Part print with two shaded views. Sizes in mm from the minimum x, y, z corner. A direction names the side the tool comes from. Give positions to 0.01 mm unless a question says otherwise; leave off trailing zeros. Order: outer loops, then holes, each group sorted by start corner. A loop starts at its lowest first (then second) coordinate and runs counter-clockwise, first axis right, second up. Notation, with made-up numbers: (-28.5, 16.25) -> (4.5, 16.25) arc R15 ccw to (4.5, 42.25) -> close; hole circle Ø10 at (85.25, -30.5). An arc over 180 degrees is marked (long way). Write item = value, one per line. Start each with the question number.
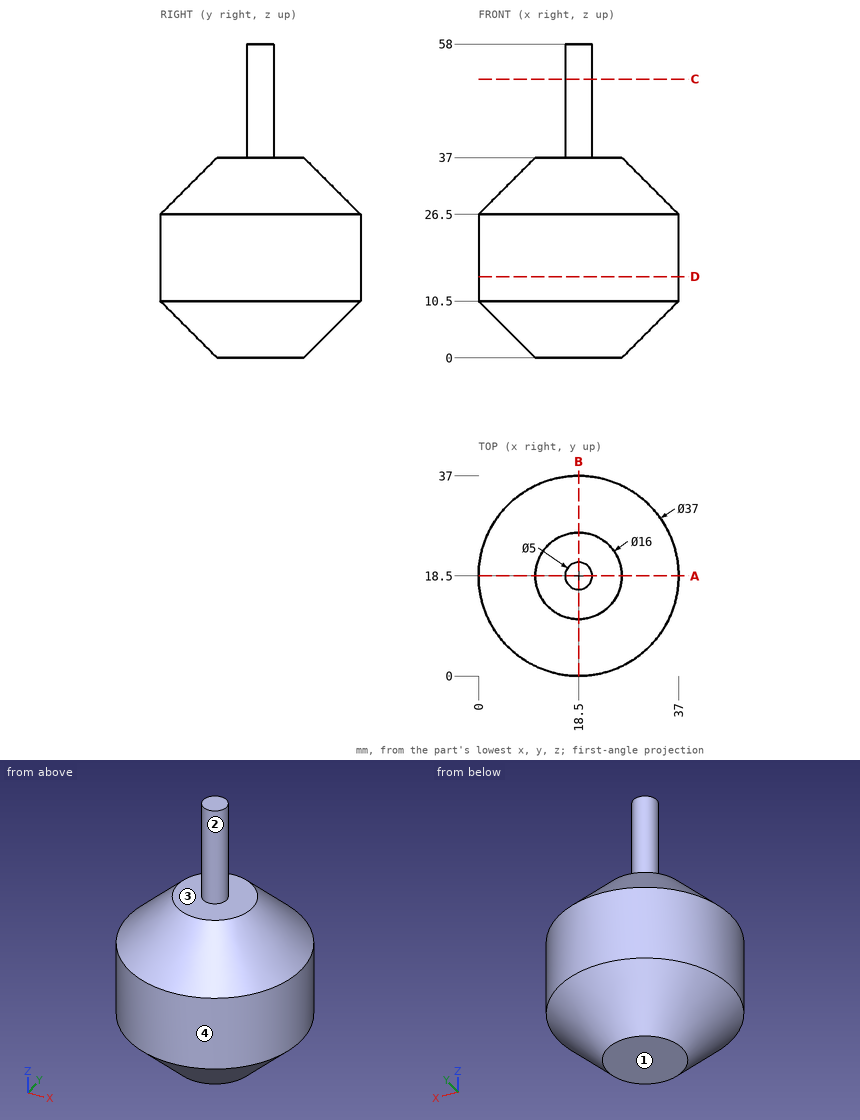
(1) Cut at C-C, the plane z = 51.5. Give the cut face in (x, y).
(2) Cut at A-A, the plane y = 18.5. Give the cut face in (x, z), plus the area to 3 significant figures.
(3) 3-axis set-ups, long thin cutter, end or side, ignore diameter. For the marked faces 1 and 2: which of +Z, -Z, +X, -X, +Y, -Y reach the whole face in a straight line?
(4) Wall check: line 1 (Y direction, x = 18, z = 11); line 2 (Z direction, x = 16.5, y = 23.5); line 3 (Z direction, x = 33, y = 27.5). Give the ranges that are in metal, low to high. Write a range as [from, to].
(5) Flat gauge pins, fed straight in: P1, Ø6, axis at x = 25, y = 31.5, coming from the +Z side; P2, Ø8, axis at x = 6, y = 4, coming from the -Z side; P3, Ø1.5, axis at x = 11, y = 20.5, coming from the +Z side. Where does each tip first touch, or does it go through?
(6) Cut at D-D, the plane z = 15. Give the cut face in (x, y).
(7) Mould opens along X. For the marked faces 3 and 4 say: released by +X, released by -X, zero draft, split by the parting line, or undercut.
Results:
q1.outline = circle Ø5 at (18.5, 18.5)
q2.outline = (0, 10.5) -> (10.5, 0) -> (26.5, 0) -> (37, 10.5) -> (37, 26.5) -> (26.5, 37) -> (21, 37) -> (21, 58) -> (16, 58) -> (16, 37) -> (10.5, 37) -> (0, 26.5) -> close
q2.area = 1,250 mm2
q3.face_1 = -Z, +X, -X, +Y, -Y
q3.face_2 = +Z
q4.line_1 = [0.01, 36.99]
q4.line_2 = [0, 37]
q4.line_3 = [9.07, 27.93]
q5.P1 = 33.47
q5.P2 = 7.14
q5.P3 = 37
q6.outline = circle Ø37 at (18.5, 18.5)
q7.face_3 = zero draft
q7.face_4 = split by the parting line
